Check sheet for the drawn part. Datum: minimum x, y, z corner. Units: mm. Round coordinates to 2 decimals unless told otherwise and drop trailing zeros. Write each loop counter-clockwise with the first axis right and the second up, starting at its lowest first coordinate (ties: lowest second). Pieces come first, ordered by that corner, then holes. Notation, with made-up numbers: M 55,87.25 L 86,87.25 A17 ccw 86,111.25 Z; hole C -27,35.5 d4. An arc over 180 degrees is marked long. One line per item, written item: value.
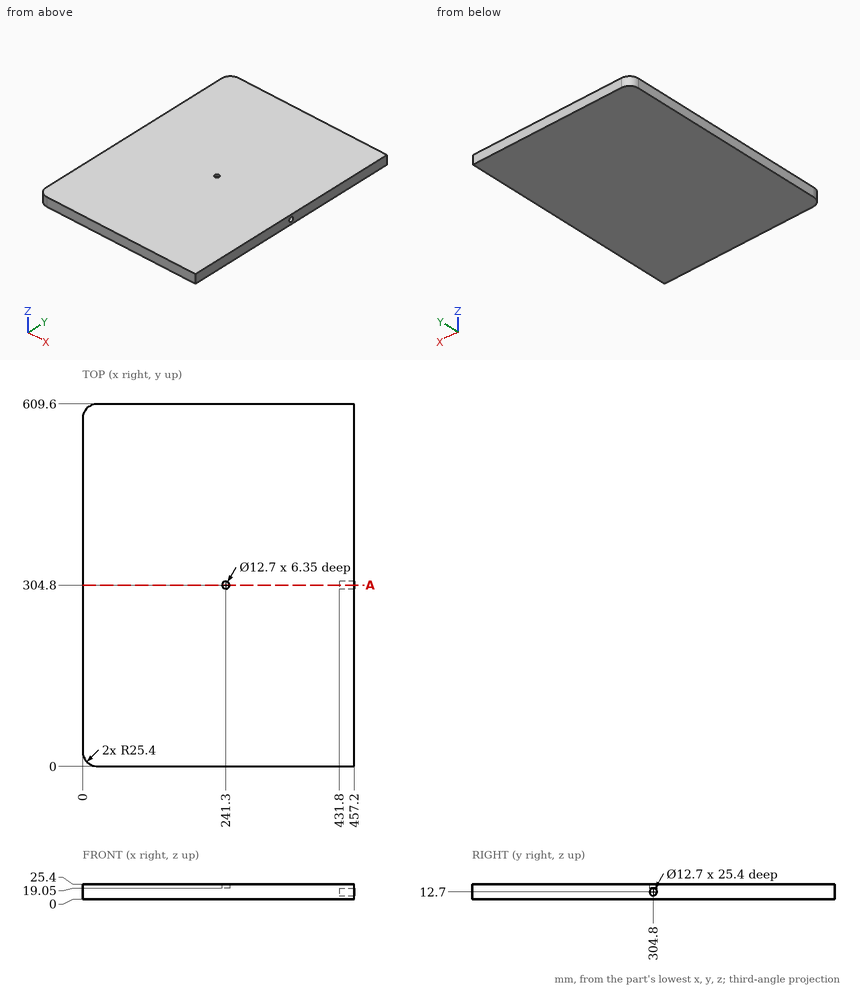
Q1. Sectioned sample at A-A on y = 304.8. Enter the section's corners in (x, z).
Completed:
outline: M 0,0 L 457.2,0 L 457.2,6.35 L 431.8,6.35 L 431.8,19.05 L 457.2,19.05 L 457.2,25.4 L 247.65,25.4 L 247.65,19.05 L 234.95,19.05 L 234.95,25.4 L 0,25.4 Z
Q2. Scan lines: line 1 (X direction, y = 304.8, z = 20.75); line 2 (Z direction, x = 450, y = 304); line 3 (Y direction, x = 241.3, z = 22.75). Record each from-to range of solid material in increasing order. Write a range as [from, to].
Completed:
line 1: [0, 234.95], [247.65, 457.2]
line 2: [0, 6.4], [19, 25.4]
line 3: [0, 298.45], [311.15, 609.6]
Q3. Depth check by flat-ended pin: P1, Ø4, axis at x = 242.5, y = 305.5, coming from the +Z side. Enter the tip coordinate at first touch or a pass-through.
Completed:
P1: z = 19.05
